```python
from build123d import *

# Parameters (mm, degrees)
SKETCH1_W                 = 80
SKETCH1_H                 = 80
SKETCH1_R                 = 14.3129
BOSS_EXTRUDE1_DEPTH       = 12.7
FILLET1_R                 = 10
CUT_EXTRUDE1_REACH        = 59.977
CUT_EXTRUDE2_REACH        = 75.221
CUT_EXTRUDE2_END_RADIUS   = 14.3129
SKETCH3_R                 = 2.665
FILLET2_R                 = 5
CUT_EXTRUDE3_REACH        = 59.977
SKETCH4_R                 = 2.665
CIRPATTERN1_COUNT         = 3
CIRPATTERN1_ANGLE         = 180
FILLET3_R                 = 5
CIRPATTERN2_COUNT         = 3
CIRPATTERN2_ANGLE         = 180
M5X0_8_TAPPED_HOLE1_D     = 4.2
M5X0_8_TAPPED_HOLE1_DEPTH = 6.35
M5X0_8_TAPPED_HOLE1_TIP   = 1.2618073


with BuildPart() as part:
    # Sketch1 → Boss-Extrude1 (new body)
    with BuildSketch(Plane(origin=(0, 0, 0), x_dir=(1, 0, 0), z_dir=(0, 1, 0))):
        Rectangle(SKETCH1_W, SKETCH1_H)
        with Locations(Location((0, 0, 0), (0, 0, 270))):
            Circle(SKETCH1_R, mode=Mode.SUBTRACT)
    extrude(amount=BOSS_EXTRUDE1_DEPTH)

    # Fillet1
    fillet1_edges = [part.edges().sort_by_distance(p)[0] for p in [
        (40, 6.35, 40),
        (-40, 6.35, 40),
        (-40, 6.35, -40),
        (40, 6.35, -40),
    ]]
    fillet(fillet1_edges, radius=FILLET1_R)

    # Sketch2 → Cut-Extrude1 (cut, up to next)
    with BuildSketch(Plane(origin=(0, 12.7, 0), x_dir=(1, 0, 0), z_dir=(0, 1, 0)), mode=Mode.PRIVATE) as cut_extrude1_sk1:
        with BuildLine():
            ThreePointArc((40, 25), (28.556310856, 16.443689144), (20, 5))
            Line((20, 5), (20, 0))
            Line((20, 0), (40, 0))
            Line((40, 0), (40, 25))
        make_face()
    cut_extrude1_tool1 = extrude(cut_extrude1_sk1.sketch, amount=-CUT_EXTRUDE1_REACH, mode=Mode.PRIVATE) & part.part
    # Sketch2 → Cut-Extrude1 (cut, up to next)
    with BuildSketch(Plane(origin=(0, 12.7, 0), x_dir=(1, 0, 0), z_dir=(0, 1, 0)), mode=Mode.PRIVATE) as cut_extrude1_sk2:
        with BuildLine():
            Line((40, 0), (20, 0))
            Line((20, 0), (20, -5))
            ThreePointArc((20, -5), (28.556310856, -16.443689144), (40, -25))
            Line((40, -25), (40, 0))
        make_face()
    cut_extrude1_tool2 = extrude(cut_extrude1_sk2.sketch, amount=-CUT_EXTRUDE1_REACH, mode=Mode.PRIVATE) & part.part
    cut_extrude1_1 = cut_extrude1_tool1.solids().sort_by_distance((31.902516, 12.7, -9.406449))[0]
    add(cut_extrude1_1, mode=Mode.SUBTRACT)
    cut_extrude1_2 = cut_extrude1_tool2.solids().sort_by_distance((31.902516, 12.7, 9.406449))[0]
    add(cut_extrude1_2, mode=Mode.SUBTRACT)
    cut_extrude1 = cut_extrude1_1 + cut_extrude1_2  # Cut-Extrude1 as one shape, for the pattern or mirror that repeats it

    # Mirror1: Cut-Extrude1 across plane
    add(cut_extrude1.mirror(Plane(origin=(0, 0, 0), x_dir=(0, 0, 1), z_dir=(1, 0, 0))), mode=Mode.SUBTRACT)

    # Cut-Extrude2: up to this cylinder (the profile starts outside it)
    cut_extrude2_end = Plane(origin=(0, 6.35, 0), z_dir=(0, -1, 0)) * Cylinder(CUT_EXTRUDE2_END_RADIUS, 180.0678, mode=Mode.PRIVATE)
    # Sketch3 → Cut-Extrude2 (cut, up to the surface)
    with BuildSketch(Plane(origin=(20, 0, 0), x_dir=(0, 0, -1), z_dir=(1, 0, 0)), mode=Mode.PRIVATE) as cut_extrude2_sk1:
        with Locations((0, 6.35)):
            Circle(SKETCH3_R)
    cut_extrude2_tool1 = extrude(cut_extrude2_sk1.sketch, amount=-CUT_EXTRUDE2_REACH, mode=Mode.PRIVATE) - cut_extrude2_end
    cut_extrude2 = cut_extrude2_tool1.solids().sort_by_distance((20, 6.35, 0))[0]
    add(cut_extrude2, mode=Mode.SUBTRACT)

    # Fillet2
    fillet2_edges = [part.edges().sort_by_distance(p)[0] for p in [
        (20, 6.35, 5),
        (20, 6.35, -5),
        (40, 6.35, -25),
        (40, 6.35, 25),
        (-20, 6.35, -5),
        (-20, 6.35, 5),
        (-40, 6.35, 25),
        (-40, 6.35, -25),
    ]]
    fillet(fillet2_edges, radius=FILLET2_R)

    # Sketch4 → Cut-Extrude3 (cut, up to next)
    with BuildSketch(Plane(origin=(0, 12.7, 0), x_dir=(1, 0, 0), z_dir=(0, 1, 0)), mode=Mode.PRIVATE) as cut_extrude3_sk1:
        with Locations(Location((-30, 30, 0), (0, 0, 270))):
            Circle(SKETCH4_R)
    cut_extrude3_tool1 = extrude(cut_extrude3_sk1.sketch, amount=-CUT_EXTRUDE3_REACH, mode=Mode.PRIVATE) & part.part
    # Sketch4 → Cut-Extrude3 (cut, up to next)
    with BuildSketch(Plane(origin=(0, 12.7, 0), x_dir=(1, 0, 0), z_dir=(0, 1, 0)), mode=Mode.PRIVATE) as cut_extrude3_sk2:
        with Locations(Location((30, 30, 0), (0, 0, 270))):
            Circle(SKETCH4_R)
    cut_extrude3_tool2 = extrude(cut_extrude3_sk2.sketch, amount=-CUT_EXTRUDE3_REACH, mode=Mode.PRIVATE) & part.part
    # Sketch4 → Cut-Extrude3 (cut, up to next)
    with BuildSketch(Plane(origin=(0, 12.7, 0), x_dir=(1, 0, 0), z_dir=(0, 1, 0)), mode=Mode.PRIVATE) as cut_extrude3_sk3:
        with Locations(Location((30, -30, 0), (0, 0, 270))):
            Circle(SKETCH4_R)
    cut_extrude3_tool3 = extrude(cut_extrude3_sk3.sketch, amount=-CUT_EXTRUDE3_REACH, mode=Mode.PRIVATE) & part.part
    # Sketch4 → Cut-Extrude3 (cut, up to next)
    with BuildSketch(Plane(origin=(0, 12.7, 0), x_dir=(1, 0, 0), z_dir=(0, 1, 0)), mode=Mode.PRIVATE) as cut_extrude3_sk4:
        with Locations(Location((-30, -30, 0), (0, 0, 270))):
            Circle(SKETCH4_R)
    cut_extrude3_tool4 = extrude(cut_extrude3_sk4.sketch, amount=-CUT_EXTRUDE3_REACH, mode=Mode.PRIVATE) & part.part
    add(cut_extrude3_tool1.solids().sort_by_distance((-30, 12.7, -30))[0], mode=Mode.SUBTRACT)
    add(cut_extrude3_tool2.solids().sort_by_distance((30, 12.7, -30))[0], mode=Mode.SUBTRACT)
    add(cut_extrude3_tool3.solids().sort_by_distance((30, 12.7, 30))[0], mode=Mode.SUBTRACT)
    add(cut_extrude3_tool4.solids().sort_by_distance((-30, 12.7, 30))[0], mode=Mode.SUBTRACT)

    # CirPattern1: Cut-Extrude1 ×3 about axis
    cirpattern1_axis = Axis((0, 0, 0), (0, -1, 0))
    for i in range(1, CIRPATTERN1_COUNT):
        add(cut_extrude1.rotate(cirpattern1_axis, i * CIRPATTERN1_ANGLE / (CIRPATTERN1_COUNT - 1)), mode=Mode.SUBTRACT)

    # Fillet3
    fillet3_edges = [part.edges().sort_by_distance(p)[0] for p in [
        (-5, 6.35, 20),
        (5, 6.35, 20),
        (25, 6.35, 40),
        (-25, 6.35, 40),
        (-20, 6.35, 5),
        (-20, 6.35, -5),
    ]]
    fillet(fillet3_edges, radius=FILLET3_R)

    # CirPattern2: Cut-Extrude2 ×3 about axis
    cirpattern2_axis = Axis((0, 12.7, 0), (0, -1, 0))
    for i in range(1, CIRPATTERN2_COUNT):
        add(cut_extrude2.rotate(cirpattern2_axis, i * CIRPATTERN2_ANGLE / (CIRPATTERN2_COUNT - 1)), mode=Mode.SUBTRACT)

    # M5x0.8 Tapped Hole1
    with Locations(Plane(origin=(16.75, 6.35, -40), x_dir=(-1, 0, 0), z_dir=(0, 0, -1))):
        with Locations((0, 0), (33.5, 0)):
            Hole(M5X0_8_TAPPED_HOLE1_D / 2, depth=M5X0_8_TAPPED_HOLE1_DEPTH)
            with Locations((0, 0, -(M5X0_8_TAPPED_HOLE1_DEPTH + M5X0_8_TAPPED_HOLE1_TIP / 2))):  # 118° drill point
                Cone(0, M5X0_8_TAPPED_HOLE1_D / 2, M5X0_8_TAPPED_HOLE1_TIP, mode=Mode.SUBTRACT)


solid = part.part
```
Can you work these out from the model? Positions are in its coordinate system, mm. A direction names the side the tool comes from. Coordinates: 2 decimals unless noted, no trailing zeros. Order: outer loops, then holes, each group sorted by start corner. A loop starts at its lowest first (then second) coordinate and runs counter-clockwise, first axis right, second up. Notation, with made-up numbers: (18, -31.75) -> (50, -31.75) arc R20 ccw to (50, 7.25) -> close; hole circle Ø3 at (79.5, 13.25). An arc over 180 degrees is marked (long way). Write each question's results on one line, items separated by ' | '.
Item 1: If I drill on line 1 along X through (y, z) = (6.5, -30) (3 decimals); line 2 along X through (y, z) = (6.25, 31.5); line 3 along Y through (x, z) = (-16.75, -38), over which ranges is the centre line in solid material (lowest first)?
Results are:
line 1: -40 to -32.665, -27.335 to 27.335, 32.665 to 40 | line 2: -39.89 to -32.2, -27.8 to -19.16, 19.16 to 27.8, 32.2 to 39.89 | line 3: 0 to 4.25, 8.45 to 12.7
Item 2: I want a section at C-C, the plane x = 35. Write out the boundary of the cut face in (y, z).
Results are:
outline: (0, -38.66) -> (12.7, -38.66) -> (12.7, -21.88) -> (0, -21.88) -> close; (0, 21.88) -> (12.7, 21.88) -> (12.7, 38.66) -> (0, 38.66) -> close
Item 3: If we mould it in two halves opening along X, with no side actions, what happens to faces 6 (the face through (40, 6, -29)), 7 (the face through (-39.35, 6.26, -25.41)), 8 (the face through (-2.115, 4.728, 17.073))? For each: +X half, -X half, draft (parallel to the pull), parting line (faces both ways), or undercut.
Results are:
face 6: +X half | face 7: -X half | face 8: undercut
Item 4: I want a section at D-D, the plane z = -1. Write out the boundary of the cut face in (x, y), then the cut area to 3 significant figures.
Results are:
outline: (-20, 0) -> (-14.28, 0) -> (-14.28, 3.88) -> (-20, 3.88) -> close; (-20, 8.82) -> (-14.28, 8.82) -> (-14.28, 12.7) -> (-20, 12.7) -> close; (14.28, 0) -> (20, 0) -> (20, 3.88) -> (14.28, 3.88) -> close; (14.28, 8.82) -> (20, 8.82) -> (20, 12.7) -> (14.28, 12.7) -> close | area: 88.8 mm²
Item 5: I want a section at B-B, the plane z = -13. Write out the boundary of the cut face in (x, y), then the cut area to 3 significant figures.
Results are:
outline: (-25.42, 0) -> (-5.99, 0) -> (-5.99, 12.7) -> (-25.42, 12.7) -> close; (5.99, 0) -> (25.42, 0) -> (25.42, 12.7) -> (5.99, 12.7) -> close | area: 494 mm²
Item 6: Which directions (+Z, -Z, +X, -X, +Y, -Y) give clear straight access to the entire face, cutting with the end or side of a thin tool? Please do faces 1 (the face through (40, 6, 29)), 2 (the face through (-25.41, 6.26, 39.35)), 3 (the face through (-27.96, 6.44, -15.84)), 4 (the face through (20.177, 6.261, -5.009)), 5 (the face through (-14.747, 6.981, -36.781)).
Results are:
face 1: +Z, -Z, +X, +Y, -Y | face 2: +Z, +Y, -Y | face 3: -X, +Y, -Y | face 4: +X, +Y, -Y | face 5: -Z
Item 7: I'm going to push flat-ended pins straight in: pin 1 Ø6 at (x, y) = (-15, 4.5) entering from +Z; pin 2 Ø4 at (y, z) = (3, -22) entering from +X; pin 3 Ø5 at (x, z) = (30, 30) entering from +Y; pin 4 Ø1 at (y, z) = (7.5, -18.5) entering from -X. Where does each tip first touch, or does it pass through?
Results are:
pin 1: z = 30.18 | pin 2: x = 38.16 | pin 3: through | pin 4: x = -31.31
Item 8: I want a section at A-A, the plane x = 0. Write out the boundary of the cut face in (y, z) (3 decimals).
Results are:
outline: (0, -40) -> (12.7, -40) -> (12.7, -14.313) -> (0, -14.313) -> close; (0, 14.313) -> (3.685, 14.313) -> (3.685, 20) -> (0, 20) -> close; (9.015, 14.313) -> (12.7, 14.313) -> (12.7, 20) -> (9.015, 20) -> close
